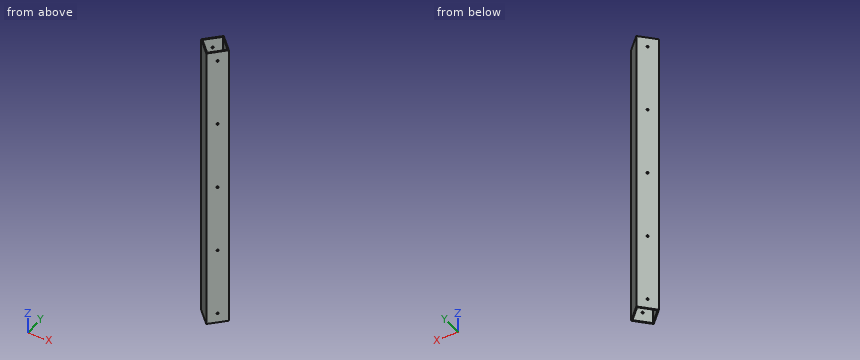
```python
from build123d import *

# Parameters (mm, degrees)
EXTRUDE_1_DEPTH     = 300
SKETCH_2_R          = 1
CUT_EXTRUDE_1_DEPTH = 31


with BuildPart() as part:
    # 草图1 → 凸台-拉伸1 (new body)
    with BuildSketch(Plane.XY):
        Polygon((14.142135624, 0), (0, 14.142135624), (-14.142135624, 0), (0, -14.142135624), align=None)
        Polygon((12.727922061, 0), (0, 12.727922061), (-12.727922061, 0), (0, -12.727922061), align=None, mode=Mode.SUBTRACT)
    extrude(amount=EXTRUDE_1_DEPTH)

    # 草图2 → 切除-拉伸1 (cut, through all)
    with BuildSketch(Plane(origin=(7.071067812, -7.071067812, 0), x_dir=(0, 0, -1), z_dir=(0.707106781, -0.707106781, 0))):
        with Locations((-290, 0)):
            Circle(SKETCH_2_R)
        with Locations((-220, 0)):
            Circle(SKETCH_2_R)
        with Locations((-150, 0)):
            Circle(SKETCH_2_R)
        with Locations((-80, 0)):
            Circle(SKETCH_2_R)
        with Locations((-10, 0)):
            Circle(SKETCH_2_R)
    extrude(amount=-CUT_EXTRUDE_1_DEPTH, mode=Mode.SUBTRACT)


solid = part.part
```
Input: part model. Units: mm. Frame: model coordinates. Coordinates: 2 decimals unless noted, no trailing zeros. Loops run counter-clockwise (first coordinate to the right, second up) from the corner with the lowest first, then second, coordinate; pieces in that order, holes last.
Q1. Line query: line 1 along Y through (x, z) = (-1.25, 209); line 2 along X through (y, z) = (4.5, 278); line 3 along Y through (x, z) = (-8.25, 149.5). Output: solid intervals per line, ascending.
Results are:
line 1: y = -12.89 to -11.48, 11.48 to 12.89
line 2: x = -9.64 to -8.23, 8.23 to 9.64
line 3: y = -5.89 to -4.48, 4.48 to 5.89
Q2. Section B-B, the plane z = 142. Return the cut outline in (x, y).
Results are:
outline: (-14.14, 0) - (0, -14.14) - (14.14, 0) - (0, 14.14) - close; hole (-12.73, 0) - (0, -12.73) - (12.73, 0) - (0, 12.73) - close
Q3. Section C-C, the plane x = 2.75. Return the cut outline in (y, z), and give its area (3 significant figures).
Results are:
outline: (-11.39, 0) - (-9.98, 0) - (-9.98, 300) - (-11.39, 300) - close; (9.98, 0) - (11.39, 0) - (11.39, 300) - (9.98, 300) - close
area: 849 mm2
Q4. Section A-A, the plane y = -3. Return the cut outline in (x, z).
Results are:
outline: (-11.14, 0) - (-9.73, 0) - (-9.73, 300) - (-11.14, 300) - close; (9.73, 0) - (11.14, 0) - (11.14, 300) - (9.73, 300) - close
Q5. Contact query for flat-ended pins moving along their axis: pin 1 (12 mm diameter, centred on x = -5, y = 1, fed in from +Z); pin 2 (10 mm diameter, centred on y = -8.5, z = 77, fed in from -X); pin 3 (1 mm diameter, centred on x = -6, z = 175.5, fed in from -Y); pin 4 (1 mm diameter, centred on x = -1, z = 234, fed in from +Y). Output: stop coordinate, or through.
Results are:
pin 1: stops at z = 300
pin 2: stops at x = -10.64
pin 3: stops at y = -8.64
pin 4: stops at y = 13.64
